from build123d import *

# Parameters (mm, degrees)
SKETCH1_R           = 11.684
BOSS_EXTRUDE1_DEPTH = 12.7
BOSS_EXTRUDE2_START = 12.7
SKETCH1_3_R         = 11.684
BOSS_EXTRUDE2_DEPTH = 45.72
SKETCH1_4_W         = 15.24
SKETCH1_4_H         = 6.35
BOSS_EXTRUDE3_DEPTH = 19.304
BOSS_EXTRUDE5_START = 39.116
SKETCH1_5_W         = 15.24
SKETCH1_5_H         = 6.35
BOSS_EXTRUDE5_DEPTH = 19.304


with BuildPart() as part:
    # Sketch1 → Boss-Extrude1 (new body)
    with BuildSketch(Plane.XY):
        with BuildLine():
            Line((-10.16, 0), (0, 0))
            Line((0, 0), (0, 6.35))
            Line((0, 6.35), (0, 25.4))
            Line((0, 25.4), (-30.48, 25.4))
            Line((-30.48, 25.4), (-30.48, 20.32))
            ThreePointArc((-30.48, 20.32), (-44.848409794, -14.368409794), (-10.16, 0))
        make_face()
        with Locations((-30.48, 0)):
            Circle(SKETCH1_R, mode=Mode.SUBTRACT)
        with BuildLine():
            Line((-30.48, 25.4), (0, 25.4))
            Line((0, 25.4), (0, 33.02))
            Line((0, 33.02), (10.16, 33.02))
            Line((10.16, 33.02), (22.86, 45.72))
            Line((22.86, 45.72), (22.86, 66.04))
            Line((22.86, 66.04), (10.16, 78.74))
            Line((10.16, 78.74), (10.16, 66.04))
            ThreePointArc((10.16, 66.04), (-15.24, 40.64), (-40.64, 66.04))
            Line((-40.64, 66.04), (-40.64, 78.74))
            Line((-40.64, 78.74), (-53.34, 66.04))
            Line((-53.34, 66.04), (-53.34, 45.72))
            Line((-53.34, 45.72), (-40.64, 33.02))
            Line((-40.64, 33.02), (-30.48, 33.02))
            Line((-30.48, 33.02), (-30.48, 25.4))
        make_face()
    extrude(amount=BOSS_EXTRUDE1_DEPTH)

    # Sketch1<3> → Boss-Extrude2 (add)
    with BuildSketch(Plane.XY.offset(BOSS_EXTRUDE2_START)):
        with BuildLine():
            Line((-30.48, 20.32), (-30.48, 25.4))
            Line((-30.48, 25.4), (0, 25.4))
            Line((0, 25.4), (0, 0))
            Line((0, 0), (-10.16, 0))
            ThreePointArc((-10.16, 0), (-44.848409794, -14.368409794), (-30.48, 20.32))
        make_face()
        with Locations((-30.48, 0)):
            Circle(SKETCH1_3_R, mode=Mode.SUBTRACT)
    extrude(amount=BOSS_EXTRUDE2_DEPTH)

    # Sketch1<4> → Boss-Extrude3 (add)
    with BuildSketch(Plane.XY):
        with Locations((7.62, 3.175)):
            Rectangle(SKETCH1_4_W, SKETCH1_4_H)
    extrude(amount=BOSS_EXTRUDE3_DEPTH)

    # Sketch1<5> → Boss-Extrude5 (add)
    with BuildSketch(Plane.XY.offset(BOSS_EXTRUDE5_START)):
        with Locations((7.62, 3.175)):
            Rectangle(SKETCH1_5_W, SKETCH1_5_H)
    extrude(amount=BOSS_EXTRUDE5_DEPTH)


solid = part.part
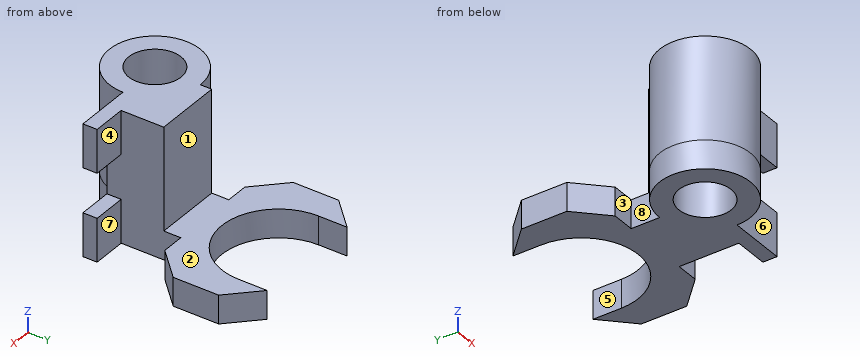
The listing builds one solid part. Answer for the finished solid, in the listing's coordinates (mm). Face numbers are marked on the shaded views. A direction names the side the tool comes from. Round coordinates to 2 decimals unless told otherwise and drop trailing zeros. Write each loop counter-clockwise with the first axis right and the second up, starting at its lowest first coordinate (ties: lowest second). Pieces come first, ordered by that corner, then holes. Notation, with made-up numbers: M 86.25,-29 L 90.25,-29 A24 cw 90.25,4 Z; hole C 56,-14 d3. An arc over 180 degrees is marked long. Write each question's results on one line, items separated by ' | '. Start each with the question number.
(1) Find the intervals of material crossed by line 1 (Y direction, x = -30, z = 33); line 2 (Y direction, x = -38, z = 7.5); line 3 (Y direction, x = -4, z = 55.5), in increasing order.
(2) Each of these flat-tipped pins is pushed along its axis until it touches: P1, Ø1.5, axis at y = -0.5, z = 7, coming from the +X side; P2, Ø8, axis at x = 10, y = 60, coming from the +Z side; P3, Ø4.5, axis at x = 7.5, z = 52.5, coming from the +Y side. Where does it stop, or does it pass through?
(3) The part is cut by section C-C, the plane x = -25. Write down the section's boundary in (y, z), and give its area (3 significant figures).
(4) The part is cut by section B-B, the plane y = 58. Write down the section's boundary in (x, z).
(5) Determine the mould class of the marked faces 1, 2 and 3 for opening direction Y: +Y half, -Y half, draft (parallel to the pull), parting line (faces both ways), or undercut.
(6) For the marked faces 4, 5, 6, 7 and 8, determine the directions among +Z, -Z, +X, -X, +Y, -Y from which every point of the face is accessible in a straight line to the end or side of a thin tool.
(7) The part is cut by section D-D, the plane x = -15.24. Write down the section's boundary in (y, z), and give its area (3 significant figures).
(8) The part is cut by section A-A, the plane z = 8. Write down the section's boundary in (x, y).
Worked answers:
1) line 1: y = -20.31 to -11.67, 11.67 to 25.4 | line 2: y = -18.88 to -8.94, 8.94 to 18.88, 33.02 to 54.76 | line 3: y = 0 to 25.4
2) P1: stops at x = 15.24 | P2: stops at z = 12.7 | P3: stops at y = 6.35
3) outline: M -19.57,0 L -10.32,0 L -10.32,58.42 L -19.57,58.42 Z; M 10.32,0 L 42.59,0 L 42.59,12.7 L 25.4,12.7 L 25.4,58.42 L 10.32,58.42 Z | area: 1,640 mm²
4) outline: M -53.34,0 L -39.33,0 L -39.33,12.7 L -53.34,12.7 Z; M 8.85,0 L 22.86,0 L 22.86,12.7 L 8.85,12.7 Z
5) face 1: +Y half | face 2: draft | face 3: undercut
6) face 4: +Z, -Z, +X, +Y | face 5: +Z, -Z, +Y | face 6: +Z, -Z, +X, -Y | face 7: +Z, -Z, +X | face 8: +Z, -Z, -X
7) outline: M -13.44,0 L 40.64,0 L 40.64,12.7 L 25.4,12.7 L 25.4,58.42 L -13.44,58.42 Z | area: 2,460 mm²
8) outline: M -53.34,45.72 L -40.64,33.02 L -30.48,33.02 L -30.48,20.32 A20.32 ccw long -10.16,0 L 15.24,0 L 15.24,6.35 L 0,6.35 L 0,33.02 L 10.16,33.02 L 22.86,45.72 L 22.86,66.04 L 10.16,78.74 L 10.16,66.04 A25.4 cw -40.64,66.04 L -40.64,78.74 L -53.34,66.04 Z; hole C -30.48,0 d23.37
